The model under review builds one solid part; all positions refer to its coordinate system, in mm. A direction names the side the tool comes from. Give positions to 0.01 mm unless a question says otherwise; leave off trailing zeros. Order: outer loops, then holes, each group sorted by start corner. A loop starts at its lowest first (then second) coordinate and runs counter-clockwise, first axis right, second up. Notation, with made-up numbers: (39, 2) - (81, 2) arc R17 ccw to (81, 30) - close; hole circle Ø8 at (12, 0). An arc over 180 degrees is marked (long way). Use CSV: the item, a comma, the result in double quotes.
```python
from build123d import *

# Parameters (mm, degrees)
F0_R      = 76.650002
F1_DEPTH  = 49.022
F2_R      = 65.6775
F3_DEPTH  = 93.98
F4_R      = 46.85452
F5_DEPTH  = 130.302
F6_R      = 2.879966
F6_R_2    = 2.810701
F6_R_3    = 3.469715
F6_R_4    = 3.981124
F7_DEPTH  = 80.264
F8_R      = 3.234533
F8_R_2    = 3.947979
F8_R_3    = 4.769434
F8_R_4    = 4.236935
F8_R_5    = 3.405214
F9_DEPTH  = 121.666
F10_R     = 4.825919
F11_DEPTH = 159.512


with BuildPart() as f1:
    # F0 (on Top) → F1 (new body)
    with BuildSketch(Plane.XY):
        Circle(F0_R)
    extrude(amount=F1_DEPTH)

    # F2 (on Top) → F3 (join)
    with BuildSketch(Plane.XY):
        Circle(F2_R)
    extrude(amount=F3_DEPTH)

    # F4 (on Top) → F5 (join)
    with BuildSketch(Plane.XY):
        Circle(F4_R)
    extrude(amount=F5_DEPTH)

    # F6 (on Top) → F7 (join)
    with BuildSketch(Plane.XY):
        with Locations((-71.895994, 0)):
            Circle(F6_R)
        with Locations((71.639679, 0)):
            Circle(F6_R_2)
        with Locations((0, 72.152309)):
            Circle(F6_R_3)
        with Locations((0, -71.383364)):
            Circle(F6_R_4)
    extrude(amount=F7_DEPTH)

    # F8 (on Top) → F9 (join)
    with BuildSketch(Plane.XY):
        with Locations((-56.260858, 0)):
            Circle(F8_R)
        with Locations((55.748228, 0)):
            Circle(F8_R_2)
        with Locations((0, -56.004543)):
            Circle(F8_R_3)
        with Locations((0, 55.491913)):
            Circle(F8_R_4)
        Circle(F8_R_5)
    extrude(amount=F9_DEPTH)

    # F10 (on Top) → F11 (join)
    with BuildSketch(Plane.XY):
        Circle(F10_R)
    extrude(amount=F11_DEPTH)


solid = f1.part
```
Item 1: Take a section at C-C, the plane z = 41.5. Give the boundary of the cut face in (x, y).
Results list:
outline,"circle Ø153.3 at (0, 0)"
Item 2: Clearance check with flat-ended pins moving along their axes: pin 1 (10 mm diameter, centred on x = -37, z = 30, fed in from -Y); pin 2 (10 mm diameter, centred on y = -38.5, z = 32, fed in from +X); pin 3 (8 mm diameter, centred on x = 26.5, y = -39.5, fed in from +Z); pin 4 (8 mm diameter, centred on x = -29, y = 20, fed in from -Z). State where each tip first meets the part, or that it passes through.
Results list:
pin 1,"stops at y = -69.65"
pin 2,"stops at x = 68.94"
pin 3,"stops at z = 130.3"
pin 4,"stops at z = 0"
Item 3: Tool access review of faces 4 (the face through (0, -56, 121.666)), 5 (the face through (56, 0, 121.666)), 6 (the face through (-10.16, -45.74, 111.89)): name each direction out of +Z, -Z, +X, -X, +Y, -Y from which nothing blocks a thin tool from reaching the whole face with its end or side.
Results list:
face 4,"+Z, +X, -X, -Y"
face 5,"+Z, +X, +Y, -Y"
face 6,"+Z"
Item 4: Take a section at D-D, the plane x = -22.5. Give the boundary of the cut face in (y, z).
Results list:
outline,"(-73.27, 0) - (73.27, 0) - (73.27, 49.02) - (61.7, 49.02) - (61.7, 93.98) - (41.1, 93.98) - (41.1, 130.3) - (-41.1, 130.3) - (-41.1, 93.98) - (-61.7, 93.98) - (-61.7, 49.02) - (-73.27, 49.02) - close"
Item 5: Mouldability with a two-part tool opening along X and no side actions: class faces 1 (the face through (51.804, 0.174, 107.629)), 2 (the face through (0, 56, 121.666)), 3 (the face through (70.805, -29.357, 24.168)) as pulls with the +X half, pulls with the -X half, needs draft (parallel to the pull), parting line crosses it, or undercut.
Results list:
face 1,"undercut"
face 2,"needs draft"
face 3,"parting line crosses it"
Item 6: Wall thickness on L1, parallel to Z at x = 16, y = 32.5; L2, parallel to Z at x = 47, y = -12.5; L3, parallel to Y at x = -8.5, z = 58: over which ranges is each line inside the solid? List them lowest first.
Results list:
L1,"z = 0 to 130.3"
L2,"z = 0 to 93.98"
L3,"y = -65.13 to 65.13"
